Work out the finished part from the listing and answer in its coordinate system (mm). Face numbers are marked on the shaded views. A direction names the side the tool comes from. Round coordinates to 2 decimals unless told otherwise and drop trailing zeros. Loops run counter-clockwise (first coordinate to the right, second up) from the corner with the lowest first, then second, coordinate; pieces in that order, holes last. Notation, with made-up numbers: M -20.5,10.25 L 3.5,10.25 A10 ccw 3.5,25.25 Z; hole C 22,70 d6. An arc over 180 degrees is marked long. One line per item, written item: value.
```python
from build123d import *

# Parameters (mm, degrees)
F0_W      = 95.25
F0_H      = 127
F1_DEPTH  = 23
F2_W      = 82.55
F2_H      = 114.3
F3_DEPTH  = 15
F4_W      = 64
F4_H      = 29
F5_DEPTH  = 25.4
F6_R      = 25.4
F7_R      = 12.7
F8_R      = 5.08
F9_W      = 14
F9_H      = 11
F10_DEPTH = 12.7
F11_W     = 15
F11_H     = 11
F12_DEPTH = 12.7


with BuildPart() as f1:
    # F0 (on Front) → F1 (new body)
    with BuildSketch(Plane.XZ):
        with Locations((0, 3.175)):
            Rectangle(F0_W, F0_H)
    extrude(amount=F1_DEPTH)

    # F2 (on face) → F3 (cut)
    with BuildSketch(Plane.XZ.offset(23)):
        with Locations((0, 3.175)):
            Rectangle(F2_W, F2_H)
    extrude(amount=-F3_DEPTH, mode=Mode.SUBTRACT)

    # F4 (on face) → F5 (cut)
    with BuildSketch(Plane.XZ.offset(8)):
        with Locations((0, 31.825)):
            Rectangle(F4_W, F4_H)
    extrude(amount=-F5_DEPTH, mode=Mode.SUBTRACT)

    # F6
    f6_edges = [f1.edges().sort_by_distance(p)[0] for p in [
        (-47.625, -11.5, 66.675),
        (47.625, -11.5, 66.675),
        (41.275, -15.5, 60.325),
        (-41.275, -15.5, 60.325),
    ]]
    fillet(f6_edges, radius=F6_R)

    # F7
    f7_edges = [f1.edges().sort_by_distance(p)[0] for p in [
        (-47.625, -11.5, -60.325),
        (47.625, -11.5, -60.325),
    ]]
    fillet(f7_edges, radius=F7_R)

    # F8
    f8_edges = [f1.edges().sort_by_distance(p)[0] for p in [
        (47.625, 0, -3.175),
        (40.185512, 0, 59.235512),
        (0, 0, 66.675),
        (-40.185512, 0, 59.235512),
        (-47.625, 0, -3.175),
    ]]
    fillet(f8_edges, radius=F8_R)

    # F9 (on face) → F10 (cut)
    with BuildSketch(Plane(origin=(0, 0, -60.325), x_dir=(1, 0, 0), z_dir=(0, 0, -1))):
        with Locations((13, 17.5)):
            Rectangle(F9_W, F9_H)
    extrude(amount=-F10_DEPTH, mode=Mode.SUBTRACT)

    # F11 (on face) → F12 (cut)
    with BuildSketch(Plane(origin=(0, 0, -60.325), x_dir=(1, 0, 0), z_dir=(0, 0, -1))):
        with Locations((-19.5, 17.5)):
            Rectangle(F11_W, F11_H)
    extrude(amount=-F12_DEPTH, mode=Mode.SUBTRACT)


solid = f1.part
```
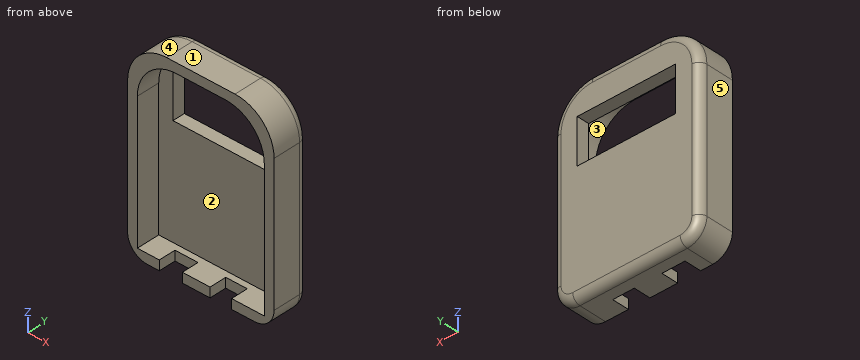
1) Each of these flat-tipped pins is pushed along its axis until it touches: pin 1 (5 mm diameter, centred on y = -19.5, z = -58, fed in from -X); pin 2 (1.9 mm diameter, centred on x = -23, z = -58, fed in from -Y); pin 3 (4 mm diameter, centred on x = 9.5, y = -3, fed in from -Z); pin 4 (1.9 mm diameter, centred on y = -15, z = -58.5, fed in from -X). Where does it stop, or does it pass through?
Check values:
pin 1: x = -44.89
pin 2: y = -12
pin 3: z = -60.32
pin 4: x = -42.85
2) Find section B-B (x = 10). Give the vertices of the cut face in (y, z) (3 decimals), then the cut area to 3 significant figures.
Check values:
outline: M -23,60.325 L -8,60.325 L -8,46.325 L 0,46.325 L 0,61.595 A5.08 ccw -5.08,66.675 L -23,66.675 Z; M -12,-60.325 L -5.08,-60.325 A5.08 ccw 0,-55.245 L 0,17.325 L -8,17.325 L -8,-53.975 L -12,-53.975 Z
area: 894 mm2
3) Find the intervals of material crossed by probe 1 along X at (y, z) = (-17.75, -31.5) (3 decimals); probe 2 along Z at (x, y) = (6, -5) (3 decimals); probe 3 along Z at (x, y) = (-3, -12.25) (3 decimals), in increasing order. Write a range as from..to.
Check values:
probe 1: -47.625..-41.275, 41.275..47.625
probe 2: -60.324..17.325, 46.325..66.674
probe 3: -60.325..-53.975, 60.325..66.675
4) The mould has two halves that part along Z. Classify the marked faces 3, 4 and 5: +Z half, -Z half, draft (parallel to the pull), parting line (faces both ways), or undercut.
Check values:
face 3: undercut
face 4: +Z half
face 5: draft
5) Find section D-D (y = -3). Give the vertices of the cut face in (x, z) (3 decimals), then the cut area to 3 significant figures.
Check values:
outline: M -47.18,-47.625 A12.255 ccw -34.925,-59.88 L 34.925,-59.88 A12.255 ccw 47.18,-47.625 L 47.18,41.275 A24.955 ccw 22.225,66.23 L -22.225,66.23 A24.955 ccw -47.18,41.275 Z; hole M -32,17.325 L 32,17.325 L 32,46.325 L -32,46.325 Z
area: 9,710 mm2
6) Find section A-A (y = -17). Give the vertices of the cut face in (x, z) (3 decimals), then the cut area to 3 significant figures.
Check values:
outline: M -47.625,-47.625 A12.7 ccw -34.925,-60.325 L -27,-60.325 L -27,-53.975 L -41.275,-53.975 L -41.275,34.925 A25.4 cw -15.875,60.325 L 15.875,60.325 A25.4 cw 41.275,34.925 L 41.275,-53.975 L 20,-53.975 L 20,-60.325 L 34.925,-60.325 A12.7 ccw 47.625,-47.625 L 47.625,41.275 A25.4 ccw 22.225,66.675 L -22.225,66.675 A25.4 ccw -47.625,41.275 Z; M -12,-60.325 L 6,-60.325 L 6,-53.975 L -12,-53.975 Z
area: 2,410 mm2
7) Find section C-C (z = 19.5). Give the vertices of the cut face in (x, y) (3 decimals), then the cut area to 3 significant figures.
Check values:
outline: M -47.625,-23 L -41.275,-23 L -41.275,-8 L -32,-8 L -32,0 L -42.545,0 A5.08 ccw -47.625,-5.08 Z; M 32,-8 L 41.275,-8 L 41.275,-23 L 47.625,-23 L 47.625,-5.08 A5.08 ccw 42.545,0 L 32,0 Z
area: 429 mm2
8) For the marked faces 1 and 2, determine the directions among +Z, -Z, +X, -X, +Y, -Y from which every point of the face is accessible in a straight line to the end or side of a thin tool.
Check values:
face 1: +Z, +X, -X, +Y, -Y
face 2: -Y
